from build123d import *

# Parameters (mm, degrees)
F0_W     = 70.698
F0_H     = 20
F1_DEPTH = 8
F2_D     = 8
F3_D     = 6.8
F4_R     = 9.99999


# Not quite as in the source:
# - a fillet or chamfer is up to 0.001 mm smaller than in the source, because OpenCascade refuses the exact size


with BuildPart() as f1:
    # F0 (on Top) → F1 (new body)
    with BuildSketch(Plane.XY):
        Rectangle(F0_W, F0_H)
    extrude(amount=-F1_DEPTH)

    # F2 (through all)
    with Locations(Plane.XY):
        with Locations((-25.349, 0)):
            Hole(F2_D / 2)

    # F3 (through all)
    with Locations(Plane.XY):
        with Locations((25.349, 0)):
            Hole(F3_D / 2)

    # F4 (radius 10 in the source; OpenCascade refuses exactly that, so slightly less here)
    f4_edges = [f1.edges().sort_by_distance(p)[0] for p in [
        (35.349, 10, -4),
        (35.349, -10, -4),
        (-35.349, 10, -4),
        (-35.349, -10, -4),
    ]]
    fillet(f4_edges, radius=F4_R)


solid = f1.part
Part model, mm, in its own coordinate system. Coordinates: 2 decimals unless noted, no trailing zeros. Order: outer loops, then holes, each group sorted by start corner. A loop starts at its lowest first (then second) coordinate and runs counter-clockwise, first axis right, second up. Notation, with made-up numbers: M 12.25,4 L 39.25,4 A12 cw 39.25,19 Z; hole C 81.5,68 d9. An arc over 180 degrees is marked long. One line per question, with ' | ' between items.
Q1. Pin check, flat tips, straight feed: P1, Ø10.5, axis at x = -25.349, y = 0, coming from the -Z side; P2, Ø1, axis at y = 4.5, z = -1.5, coming from the -X side; P3, Ø3, axis at y = -6, z = -3.5, coming from the -X side. Stop position of each tip, or through.
A:
P1: stops at z = -8 | P2: stops at x = -34.51 | P3: stops at x = -34.28
Q2. Slice it at C-C (x = 31). Give the cut face in (y, z), and give its area (3 significant figures).
A:
outline: M -8.25,-8 L 8.25,-8 L 8.25,0 L -8.25,0 Z | area: 132 mm^2
Q3. Drill centre lines: line 1 (X direction, y = 2.75, z = -2); line 2 (X direction, y = -3, z = -4.5); line 3 (Y direction, x = 25.5, z = -7.5). Where is each one in solid material? Low to high.
A:
line 1: x = -34.96 to -28.25, -22.44 to 23.35, 27.35 to 34.96 | line 2: x = -34.89 to -27.99, -22.7 to 23.75, 26.95 to 34.89 | line 3: y = -10 to -3.4, 3.4 to 10
Q4. Slice it at B-B (y = 6.5). Give the cut face in (x, z).
A:
outline: M -32.95,-8 L 32.95,-8 L 32.95,0 L -32.95,0 Z
Q5. Slice it at A-A (z = -4.75). Count the separate pieces of the cut face and the enclosed holes in it, and give its area (3 significant figures).
A:
separate pieces: 1 | enclosed holes: 2 | area: 1,240 mm^2
Q6. Two-plate mould, pull along Y, no slides. Class faces 1 (the face through (32.34, 7.15, -4.06)), 2 (the face through (32.34, -7.15, -4.06)), 3 (the face through (-29.044, -1.532, -4.056)): +Y half, -Y half, draft (parallel to the pull), parting line (faces both ways), or undercut.
A:
face 1: +Y half | face 2: -Y half | face 3: undercut
